Verification items for the finished model (mm, model axes). Face numbers are marked on the shaded views. Coordinates: 2 decimals unless noted, no trailing zeros. Order: outer loops, then holes, each group sorted by start corner. A loop starts at its lowest first (then second) coordinate and runs counter-clockwise, first axis right, second up. Notation, with made-up numbers: M 28,36 L 65,36 A19 cw 65,45 Z; hole C 86.5,-13.5 d11. An arc over 180 degrees is marked long. Answer as a JSON object with one key per item and string values. Group by question number.
(1) Mould release check, pull along X, two halves, no side actions. Record for the marked faces 1, 2, 3 and 4: released by +X, released by -X, zero draft, split by the parting line, or undercut.
(2) Cross-section at B-B (y = 4.5). Enter the section's corners in (x, z), plus the area to 3 significant figures.
(3) Cross-section at C-C (z = -28.5). Enter the section's corners in (x, y).
(4) Cross-section at A-A (x = 3.5). Enter the section's corners in (y, z), plus the area to 3 significant figures.
(5) Material ranges on line 1 (X direction, y = 7.5, z = 99); line 2 (Y direction, x = 7, z = 50); line 3 (X direction, y = -12, z = 162), recorded low to high.
(6) Cross-section at D-D (z = 115.5). Enter the section's corners in (x, y).
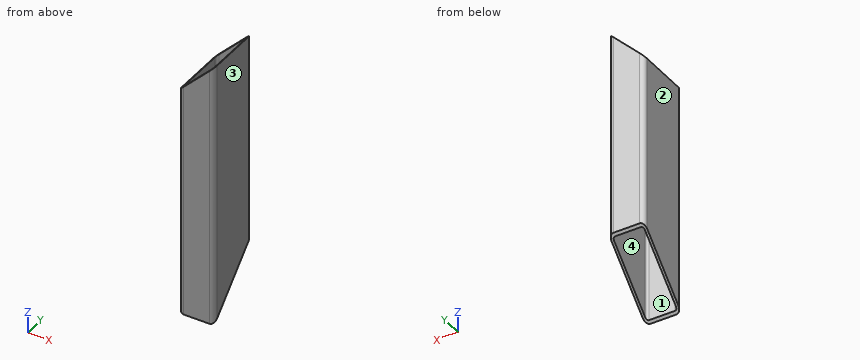
Autodesk Inventor part; units mm, degrees
ref_plane "Plano inicial" through (0, 0, -50) normal (0, 0, 1) x (1, 0, 0)
ref_plane "Plano final" through (0, 0, 175) normal (0, 0, 1) x (1, 0, 0)
ref_plane "Plano de trabalho7" through (0, -25, -50) normal (0, 0.7071, -0.7071) x (1, 0, 0)
ref_plane "Plano inicial" through (0, 0, -50) normal (0, 0, 1) x (1, 0, 0)
ref_plane "Plano final" through (0, 0, 175) normal (0, 0, 1) x (1, 0, 0)
sketch "Rascunho" plane through (0, 0, 0) normal (0, 0, 1) x (1, 0, 0)
  line L0 (-15, -21) -> (-15, 21)
  line L1 (-11, 25) -> (11, 25)
  line L2 (15, 21) -> (15, -21)
  line L3 (11, -25) -> (-11, -25)
  arc A0 (-15, -21) -> (-11, -25) centre (-11, -21) ccw
  arc A1 (15, 21) -> (11, 25) centre (11, 21) ccw
  arc A2 (-11, 25) -> (-15, 21) centre (-11, 21) ccw
  arc A3 (11, -25) -> (15, -21) centre (11, -21) ccw
  arc A4 (-11, 23) -> (-13, 21) centre (-11, 21) ccw
  line L4 (-11, 23) -> (11, 23)
  arc A5 (13, 21) -> (11, 23) centre (11, 21) ccw
  line L5 (13, 21) -> (13, -21)
  arc A6 (11, -23) -> (13, -21) centre (11, -21) ccw
  line L6 (11, -23) -> (-11, -23)
  arc A7 (-13, -21) -> (-11, -23) centre (-11, -21) ccw
  line L7 (-13, -21) -> (-13, 21)
  line L8 (0, 36.1598) -> (0, -36.1598) construction
  line L9 (-22.1598, 0) -> (22.1598, 0) construction
  dimension "d7" = 4
  dimension "d9" = 30
  dimension "d11" = 50
  dimension "d12" = 2
  dimension "d15" = 15
  dimension "d16" = 25
extrude "Corpo" add sketch "Rascunho" along normal up to surface (225 mm away) from surface at -50
sketch "Sketch3" plane through (0, 0, 0) normal (0, 0, 1) x (1, 0, 0)
  line L0 (0, 0) -> (10, 0)
ref_plane "Work Plane3" through (0, 0, 0) normal (0, -1, 0) x (1, 0, 0)
sketch "Sketch4" plane through (0, 0, 0) normal (0, -1, 0) x (1, 0, 0)
  line L0 (-2, -50) -> (12, -50)
  line L1 (-2, 175) -> (12, 175)
  dimension "d18" = 225
ref_plane "Plano de trabalho7" through (0, -25, -50) normal (0, 0.7071, -0.7071) x (1, 0, 0)
split "Dividir4" plane through (0, -25, -50) removes the side toward (0, 0.7071, -0.7071)
ref_plane "Plano de trabalho10" through (15, 0, 175) normal (-0.7071, 0, 0.7071) x (0.7071, 0, 0.7071)
split "Dividir7" plane through (15, 0, 175) removes the side toward (-0.7071, 0, 0.7071)
equation "\"d7\" = G_IR"
equation "\"d9\" = G_W"
equation "\"d11\" = G_H"
equation "\"d12\" = G_T"
equation "\"d15\" = 0.5 * d9"
equation "\"d16\" = 0.5 * d11"
equation "\"d3\" = G_L"
equation "\"G_W\" = 30"
equation "\"G_H\" = 50"
equation "\"G_T\" = 2"
equation "\"G_IR\" = 4"
equation "\"G_L\" = d18"
equation "\"G_OFFSET_END\" = 0"
equation "\"d14\" = G_OFFSET_END + B_L"
equation "\"B_L\" = 175"
properties part number "ISO 4019 - 50x30x2 - 225" material "Aço, suave"
Taken from the geometry:
{
 "1": {"face 1": "undercut", "face 2": "released by -X", "face 3": "released by +X", "face 4": "undercut"},
 "2": {"outline": "M -15,-20.5 L -13,-20.5 L -13,147 L -15,145 Z; M 13,-20.5 L 15,-20.5 L 15,175 L 13,173 Z", "area": "722 mm²"},
 "3": {"outline": "M -15,-21 A4 ccw -11,-25 L 11,-25 A4 ccw 15,-21 L 15,-3.5 L 13,-3.5 L 13,-21 A2 cw 11,-23 L -11,-23 A2 cw -13,-21 L -13,-3.5 L -15,-3.5 Z"},
 "4": {"outline": "M -25,-50 L -23,-48 L -23,163.5 L -25,163.5 Z; M 23,-2 L 25,0 L 25,163.5 L 23,163.5 Z", "area": "754 mm²"},
 "5": {"line 1": "x = -15 to -13, 13 to 15", "line 2": "y = -25 to -23, 23 to 25", "line 3": "x = 13 to 15"},
 "6": {"outline": "M -15,-21 A4 ccw -11,-25 L 11,-25 A4 ccw 15,-21 L 15,21 A4 ccw 11,25 L -11,25 A4 ccw -15,21 Z; hole M -13,-21 A2 ccw -11,-23 L 11,-23 A2 ccw 13,-21 L 13,21 A2 ccw 11,23 L -11,23 A2 ccw -13,21 Z"}
}
